Read the model definition and answer for the solid it produces. Units are mm, in the model's axes. A direction names the side the tool comes from. Give positions to 0.01 mm unless a question says otherwise; leave off trailing zeros. Loops run counter-clockwise (first coordinate to the right, second up) from the corner with the lowest first, then second, coordinate; pieces in that order, holes last. Notation, with made-up numbers: (-0.5, 2.5) - (48.5, 2.5) arc R30 ccw to (48.5, 27.5) - close; hole circle Ø8 at (4, 75.5). An arc over 180 degrees is marked (long way). Write item = value, one per line. Start each with the question number.
from build123d import *

# Parameters (mm, degrees)
EXTRUDE1_DEPTH          = 50.8
SKETCH3_W               = 60
SKETCH3_H               = 98.6
CUT_EXTRUDE1_DEPTH      = 48.5
CUT_EXTRUDE1_DEPTH_BACK = 650.5
EXTRUDE2_DEPTH          = 253.5
EXTRUDE2_DEPTH_BACK     = 253.5
EXTRUDE8_DEPTH          = 75
SKETCH4_W               = 30
SKETCH4_H               = 66
CUT_EXTRUDE2_DEPTH      = 46
LPATTERN1_COUNT         = 6
LPATTERN1_PITCH         = 90
SKETCH10_R              = 2.25
EXTRUDE7_DEPTH          = 102.6
SKETCH13_W              = 158
SKETCH13_H              = 135
SKETCH13_W_2            = 38
SKETCH13_H_2            = 15
EXTRUDE10_DEPTH         = 100
EXTRUDE10_DEPTH_BACK    = 700


with BuildPart() as part:
    # Sketch2 → Extrude1 (new body, symmetric)
    with BuildSketch(Plane.XY):
        Polygon((168.229133429, 47.5), (168.229133429, -47.5), (159.029133429, -81.83486743), (159.029133429, -520.16513257), (168.229133429, -554.5), (168.229133429, -649.5), (204.029133429, -649.5), (204.029133429, 47.5), align=None)
    extrude(amount=EXTRUDE1_DEPTH, both=True)

    # Sketch3 → Cut-Extrude1 (cut, two sides)
    with BuildSketch(Plane(origin=(0, 0, 0), x_dir=(1, 0, 0), z_dir=(0, 1, 0))) as cut_extrude1_sk:
        with Locations((172.529133429, 0)):
            Rectangle(SKETCH3_W, SKETCH3_H)
    extrude(amount=CUT_EXTRUDE1_DEPTH, mode=Mode.SUBTRACT)
    extrude(cut_extrude1_sk.sketch, amount=-CUT_EXTRUDE1_DEPTH_BACK, mode=Mode.SUBTRACT)


with BuildPart() as body_2:
    # Sketch5 → Extrude2 (new body, two sides)
    with BuildSketch(Plane(origin=(0, -301, 0), x_dir=(1, 0, 0), z_dir=(0, 1, 0))) as extrude2_sk:
        Polygon((198.029133429, 13.4125), (202.529133429, 13.4125), (202.529133429, -1.5875), (164.529133429, -1.5875), (164.529133429, 1.4125), (198.029133429, 1.4125), align=None)
    extrude(amount=EXTRUDE2_DEPTH)
    extrude(extrude2_sk.sketch, amount=-EXTRUDE2_DEPTH_BACK)

    # Sketch11 → Extrude8 (cut, symmetric)
    with BuildSketch(Plane.XY):
        Polygon((170.973907148, -47.5), (153.959133429, -111), (130.029133429, -111), (130.029133429, -11), (170.973907148, -11), align=None)
        Polygon((153.959133429, -491), (130.029133429, -491), (130.029133429, -591), (170.973907148, -591), (170.973907148, -554.5), align=None)
    extrude(amount=EXTRUDE8_DEPTH, both=True, mode=Mode.SUBTRACT)


with BuildPart() as cut_extrude2_tool:
    # Sketch4 → Cut-Extrude2 (new body, symmetric)
    with BuildSketch(Plane.XY):
        with Locations((194.029133429, -262.7)):
            Rectangle(SKETCH4_W, SKETCH4_H)
    extrude(amount=CUT_EXTRUDE2_DEPTH, both=True)


with BuildPart() as part_1:
    add(part.part)

    # Cut-Extrude2: cut by cut_extrude2_tool
    add(cut_extrude2_tool.part, mode=Mode.SUBTRACT)


with BuildPart() as body_2_1:
    add(body_2.part)

    # Cut-Extrude2: cut by cut_extrude2_tool
    add(cut_extrude2_tool.part, mode=Mode.SUBTRACT)


with BuildPart() as tapped_hole_for_8_32_helicoil1_tool:
    # Sketch34 → Tapped Hole for #8-32 Helicoil1 (revolve)
    with BuildSketch(Plane(origin=(204.029133429, -77.011124935, -7.640243296), x_dir=(0, 0, -1), z_dir=(0, 1, 0))):
        Polygon((0, 0), (0, 45), (2.1971, 45), (2.1971, 5), (2.63779, 5), (2.63779, 0), align=None)
    tapped_hole_for_8_32_helicoil1 = revolve(axis=Axis((210.379133429, -77.011124935, -7.640243296), (-1, 0, 0)))


with BuildPart() as part_2:
    add(part_1.part)

    # Tapped Hole for #8-32 Helicoil1: cut by tapped_hole_for_8_32_helicoil1_tool
    add(tapped_hole_for_8_32_helicoil1_tool.part, mode=Mode.SUBTRACT)


with BuildPart() as body_2_2:
    add(body_2_1.part)

    # Tapped Hole for #8-32 Helicoil1: cut by tapped_hole_for_8_32_helicoil1_tool
    add(tapped_hole_for_8_32_helicoil1_tool.part, mode=Mode.SUBTRACT)


with BuildPart() as lpattern1_tool:
    # LPattern1: Tapped Hole for #8-32 Helicoil1 ×6, 1 skipped
    with Locations(*[(0, -i * LPATTERN1_PITCH, 0) for i in range(1, LPATTERN1_COUNT) if i not in (2,)]):
        add(tapped_hole_for_8_32_helicoil1)


with BuildPart() as part_3:
    add(part_2.part)

    # LPattern1: cut by lpattern1_tool
    add(lpattern1_tool.part, mode=Mode.SUBTRACT)

    # Sketch10 → Extrude7 (cut, through all)
    with BuildSketch(Plane.XY.offset(50.8)):
        with Locations((192.854133429, -102.5)):
            Circle(SKETCH10_R)
        with Locations((192.854133429, -117.5)):
            Circle(SKETCH10_R)
        with Locations((192.854133429, -327.5)):
            Circle(SKETCH10_R)
        with Locations((192.854133429, -312.5)):
            Circle(SKETCH10_R)
        with Locations((192.854133429, -42.5)):
            Circle(SKETCH10_R)
        with Locations((192.854133429, -27.5)):
            Circle(SKETCH10_R)
        with Locations((192.854133429, -586.5)):
            Circle(SKETCH10_R)
        with Locations((192.854133429, -601.5)):
            Circle(SKETCH10_R)
    extrude(amount=-EXTRUDE7_DEPTH, mode=Mode.SUBTRACT)

    # Sketch13 → Extrude10 (cut, two sides)
    with BuildSketch(Plane(origin=(0, 0, 0), x_dir=(1, 0, 0), z_dir=(0, 1, 0))) as extrude10_sk:
        with Locations((183.529133429, 5.9125)):
            Rectangle(SKETCH13_W, SKETCH13_H)
        with Locations((183.529133429, 5.9125)):
            Rectangle(SKETCH13_W_2, SKETCH13_H_2, mode=Mode.SUBTRACT)
    extrude(amount=EXTRUDE10_DEPTH, mode=Mode.SUBTRACT)
    extrude(extrude10_sk.sketch, amount=-EXTRUDE10_DEPTH_BACK, mode=Mode.SUBTRACT)


with BuildPart() as body_2_3:
    add(body_2_2.part)

    # LPattern1: cut by lpattern1_tool
    add(lpattern1_tool.part, mode=Mode.SUBTRACT)


solid = body_2_3.part
1. A cutting plane is placed at A-A on y = -130. Give the vertices of the cut face in (x, z).
2. Given P1, Ø7, axis at y = -347.01, z = -7.64, coming from the -X side; P2, Ø2, axis at x = 185.5, y = -185, coming from the -Z side; P3, Ø4, axis at y = -167.5, z = -8.5, coming from the +X side; P4, Ø7.5, axis at x = 188, z = -7.5, coming from the +Y side, each flat-ended and moving along its own axis, determine where each tip first touches the part or whether it passes through.
3. Consider line 1 along Z through (x, y) = (198.5, -527); line 2 along Z through (x, y) = (185, -346); line 3 along Y through (x, z) = (201.5, -1.5). Determine where each line is inside the solid, lowest interval first. Write a range as [from, to].
4. A tool of negligible diameter and unlimited length cuts with its end or side. For faces 1 (the flat face through (202.529, -423, -6)), 2 (the flat face through (196, -295.7, -1)), 3 (the flat face through (198.029, -423, -7)), from which of +Z, -Z, +X, -X, +Y, -Y can it reach the whole face along a straight path? Write none if from no direction.
5. For a pull along Y with two mould halves and no side action, classify faces 4 (the flat face through (196, -229.7, -1)), 5 (the flat face through (193, -47.5, -1)), 6 (the flat face through (193, -554.5, -1)), 7 (the flat face through (202.529, -137, -6)) as released by +Y, released by -Y, zero draft, split by the parting line, or undercut.
6. A cutting plane is placed at B-B on y = -239.5. Give the vertices of the cut face in (x, z).
Reply:
q1.outline = (164.53, -1.41) - (198.03, -1.41) - (198.03, -13.41) - (202.53, -13.41) - (202.53, 1.59) - (164.53, 1.59) - close
q2.P1 = 198.03
q2.P2 = -1.41
q2.P3 = 202.53
q2.P4 = through
q3.line_1 = [-13.41, -9.84], [-5.44, 1.59]
q3.line_2 = [-1.41, 1.59]
q3.line_3 = [-554.5, -295.7], [-229.7, -47.5]
q4.face_1 = +Z, -Z, +X, +Y, -Y
q4.face_2 = +Z, -Z, +X
q4.face_3 = -Z, -X, +Y, -Y
q5.face_4 = undercut
q5.face_5 = released by +Y
q5.face_6 = released by -Y
q5.face_7 = zero draft
q6.outline = (164.53, -1.41) - (179.03, -1.41) - (179.03, 1.59) - (164.53, 1.59) - close
